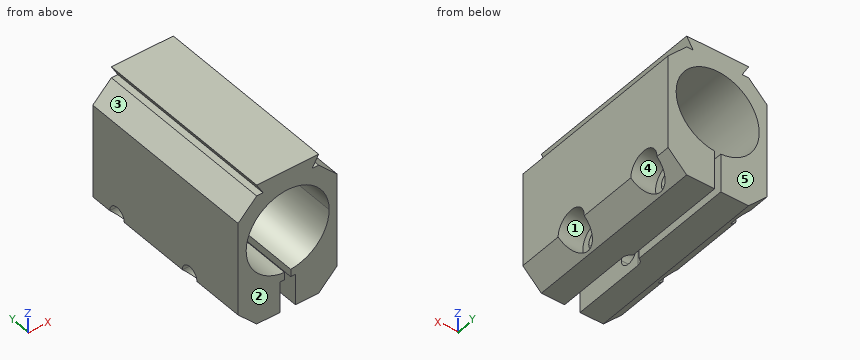
from build123d import *

# Parameters (mm, degrees)
F0_R     = 8.509
F1_DEPTH = 38.1
F3_DEPTH = 6.35
F5_DEPTH = 5.08
F6_DEPTH = 20.321
F8_DEPTH = 8.897727111


# Not quite as in the source:
# - a feature names something its author has since deleted; it is built from what else it names


with BuildPart() as f1:
    # F0 (on Front) → F1 (new body)
    with BuildSketch(Plane.XZ):
        Polygon((5.0301772846, 10.414), (-5.0301772846, 10.414), (-6.35, 10.414), (-10.16, 6.604), (-10.16, -12.5681449387), (-6.3451449387, -16.383), (6.35, -16.383), (10.16, -12.573), (10.16, 6.604), (6.35, 10.414), align=None)
        Circle(F0_R, mode=Mode.SUBTRACT)
        Polygon((6.35, 12.7), (-6.35, 12.7), (-5.0301772846, 10.414), (5.0301772846, 10.414), align=None)
    extrude(amount=F1_DEPTH)

    # F2 (on face) → F3 (cut)
    with BuildSketch(Plane(origin=(0, 0, -16.383), x_dir=(1, 0, 0), z_dir=(0, 0, -1))):
        with BuildLine():
            Line((1.5875, 38.1), (-1.5875, 38.1))
            Line((-1.5875, 38.1), (-1.5875, 22.86))
            ThreePointArc((-1.5875, 22.86), (0, 21.2725), (1.5875, 22.86))
            Line((1.5875, 22.86), (1.5875, 38.1))
        make_face()
    extrude(amount=-F3_DEPTH, mode=Mode.SUBTRACT)

    # F4 (on face) → F5 (cut)
    with BuildSketch(Plane.YZ.offset(10.16)):
        with BuildLine():
            ThreePointArc((-28.829, -12.573), (-25.4, -16.002), (-21.971, -12.573))
            Line((-21.971, -12.573), (-23.495, -12.573))
            ThreePointArc((-23.495, -12.573), (-25.4, -14.478), (-27.305, -12.573))
            Line((-27.305, -12.573), (-28.829, -12.573))
        make_face()
        with BuildLine():
            ThreePointArc((-2.921, -12.573), (-6.35, -9.144), (-9.779, -12.573))
            Line((-9.779, -12.573), (-8.255, -12.573))
            ThreePointArc((-8.255, -12.573), (-6.35, -10.668), (-4.445, -12.573))
            Line((-4.445, -12.573), (-2.921, -12.573))
        make_face()
        with BuildLine():
            Line((-8.255, -12.573), (-9.779, -12.573))
            ThreePointArc((-9.779, -12.573), (-6.35, -16.002), (-2.921, -12.573))
            Line((-2.921, -12.573), (-4.445, -12.573))
            ThreePointArc((-4.445, -12.573), (-6.35, -14.478), (-8.255, -12.573))
        make_face()
        with BuildLine():
            Line((-23.495, -12.573), (-21.971, -12.573))
            ThreePointArc((-21.971, -12.573), (-25.4, -9.144), (-28.829, -12.573))
            Line((-28.829, -12.573), (-27.305, -12.573))
            ThreePointArc((-27.305, -12.573), (-25.4, -10.668), (-23.495, -12.573))
        make_face()
    extrude(amount=-F5_DEPTH, mode=Mode.SUBTRACT)

    # F6 (cut, through all): faces of the model
    f6_faces = [f1.faces().sort_by_distance(p)[0] for p in [
        (10.16, -25.4, -11.7644928891),
        (9.3514928891, -25.4, -13.3815071109),
        (10.16, -6.35, -11.7644928891),
        (9.3514928891, -6.35, -13.3815071109),
    ]]
    extrude(f6_faces, amount=-F6_DEPTH, dir=(1, 0, 0), mode=Mode.SUBTRACT)

    # F7 (on face) → F8 (cut, up to face)
    with BuildSketch(Plane(origin=(0, 0, -16.383), x_dir=(1, 0, 0), z_dir=(0, 0, -1))):
        with BuildLine():
            Line((-0.635, 0), (0.635, 0))
            Line((0.635, 0), (0.635, 21.4050322169))
            ThreePointArc((0.635, 21.4050322169), (0, 21.2725), (-0.635, 21.4050322169))
            Line((-0.635, 21.4050322169), (-0.635, 0))
        make_face()
        with BuildLine():
            ThreePointArc((-0.635, 21.4050322169), (0, 21.2725), (0.635, 21.4050322169))
            Line((0.635, 21.4050322169), (0.635, 38.1))
            Line((0.635, 38.1), (-0.635, 38.1))
            Line((-0.635, 38.1), (-0.635, 21.4050322169))
        make_face()
    extrude(amount=-F8_DEPTH, mode=Mode.SUBTRACT)


solid = f1.part
Here's how the part is built. I have some questions about the finished solid (model axes, mm). Face numbers are marked on the shaded views. A direction names the side the tool comes from. Round coordinates to 2 decimals unless told otherwise and drop trailing zeros. Order: outer loops, then holes, each group sorted by start corner. A loop starts at its lowest first (then second) coordinate and runs counter-clockwise, first axis right, second up. Notation, with made-up numbers: M -10,-28.5 L 26,-28.5 A24 cw 26,-13.5 Z; hole C -4,-34.75 d9. An arc over 180 degrees is marked long. One line per question, with ' | ' between items.
1) Imagine slicing it at D-D, the plane x = -2.5. Count the separate pieces of the cut face and the enclosed holes in it, plus the area to 3 significant figures.
Checked values:
separate pieces: 2 | enclosed holes: 2 | area: 465 mm²
2) On a 3-axis mill with a long thin cutter (end or side, diameter ignored), from which of +Z, -Z, +X, -X, +Y, -Y can I reach the whole of each face in a straight line? I mean the marked faces 4 and 5. Say none if no direction works.
Checked values:
face 4: +X | face 5: +Z, -Z, +X, -X, +Y
3) Imagine slicing it at C-C, the plane x = 8. Write out the boundary of the cut face in (y, z).
Checked values:
outline: M -38.1,-14.73 L -28.06,-14.73 A3.43 cw long -22.74,-14.73 L -9.01,-14.73 A3.43 cw long -3.69,-14.73 L 0,-14.73 L 0,-2.9 L -38.1,-2.9 Z; M -38.1,2.9 L 0,2.9 L 0,8.76 L -38.1,8.76 Z
4) Imagine slicing it at B-B, the plane y = -20. Write out the boundary of the cut face in (x, z) (3 decimals), plus the area to 3 significant figures.
Checked values:
outline: M -10.16,-12.568 L -6.345,-16.383 L -0.635,-16.383 L -0.635,-8.485 A8.509 cw long 0.635,-8.485 L 0.635,-16.383 L 6.35,-16.383 L 10.16,-12.573 L 10.16,6.604 L 6.35,10.414 L 5.03,10.414 L 6.35,12.7 L -6.35,12.7 L -5.03,10.414 L -6.35,10.414 L -10.16,6.604 Z | area: 304 mm²
5) Imagine slicing it at A-A, the plane z = 7.25. Write out the boundary of the cut face in (x, y), plus the area to 3 significant figures.
Checked values:
outline: M -9.51,-38.1 L -4.45,-38.1 L -4.45,0 L -9.51,0 Z; M 4.45,-38.1 L 9.51,-38.1 L 9.51,0 L 4.45,0 Z | area: 386 mm²
6) I need wall thicknesses on line 1 (Y direction, x = -7, z = -14); line 2 (Y direction, x = 6.5, z = -11.5); line 3 (Z direction, x = 1.75, y = -26). Which ranges of each line are inside material? Lowest first, please.
Checked values:
line 1: y = -38.1 to -26.66, -24.14 to -7.61, -5.09 to 0 | line 2: y = -38.1 to -28.66, -22.14 to -9.61, -3.09 to 0 | line 3: z = -16.38 to -14.38, -10.76 to -8.33, 8.33 to 12.7
7) We'd pull the mould along Y, two halves only. Please class the marked faces 1, 2 and 3: released by +Y, released by -Y, zero draft, split by the parting line, or undercut.
Checked values:
face 1: undercut | face 2: released by -Y | face 3: zero draft
8) I'm going to push flat-ended pins straight in: pin 1 Ø2 at (y, z) = (-25, -13) entering from +X; pin 2 Ø4 at (y, z) = (-25.4, -12.573) entering from +X; pin 3 Ø1 at (x, y) = (-1, -31.5) entering from -Z; pin 4 Ø1.9 at (y, z) = (-28, -14) entering from -X. Where does each tip first touch, or does it pass through?
Checked values:
pin 1: passes through | pin 2: stops at x = 5.08 | pin 3: stops at z = -10.03 | pin 4: stops at x = -9.68
